from build123d import *

# Parameters (mm, degrees)
BOSS_EXTRUDE1_DEPTH = 46
CUT_EXTRUDE1_REACH  = 48
SKETCH2_R           = 1.65
SKETCH3_R           = 1.65
CUT_EXTRUDE2_DEPTH  = 5


with BuildPart() as part:
    # Sketch1 → Boss-Extrude1 (new body)
    with BuildSketch(Plane(origin=(-73, 0, 0), x_dir=(0, 0, 1), z_dir=(0, 1, 0))):
        Polygon((82, 10.55666667), (90, 8.18333333), (90, -9), (82, -9), align=None)
    extrude(amount=BOSS_EXTRUDE1_DEPTH)

    # Sketch2 → Cut-Extrude1 (cut, up to next)
    with BuildSketch(Plane.XZ, mode=Mode.PRIVATE) as cut_extrude1_sk1:
        with Locations((-73.41, 86)):
            Circle(SKETCH2_R)
    cut_extrude1_tool1 = extrude(cut_extrude1_sk1.sketch, amount=-CUT_EXTRUDE1_REACH, mode=Mode.PRIVATE) & part.part
    add(cut_extrude1_tool1.solids().sort_by_distance((-73.41, 0, 86))[0], mode=Mode.SUBTRACT)

    # Sketch3 → Cut-Extrude2 (cut)
    with BuildSketch(Plane.ZY.offset(82)):
        with Locations((86, 34.5)):
            Circle(SKETCH3_R)
        with Locations((86, 11.5)):
            Circle(SKETCH3_R)
    extrude(amount=-CUT_EXTRUDE2_DEPTH, mode=Mode.SUBTRACT)


solid = part.part
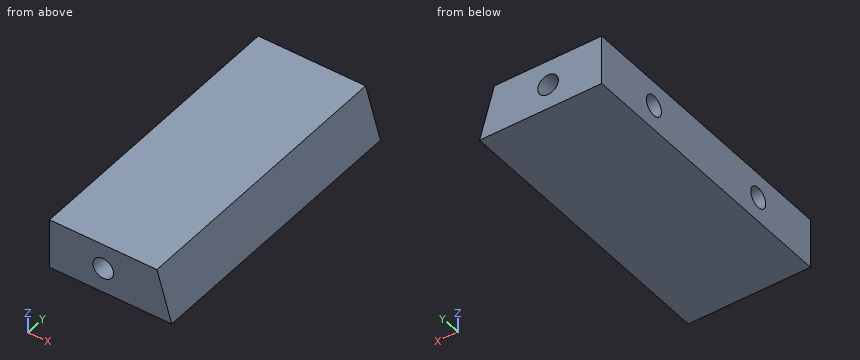
Part model, mm, in its own coordinate system. Coordinates: 2 decimals unless noted, no trailing zeros. Loops run counter-clockwise (first coordinate to the right, second up) from the corner with the lowest first, then second, coordinate; pieces in that order, holes last. Notation, with made-up numbers: (9, 37) -> (24, 37) arc R11 cw to (24, 43) -> close; hole circle Ø11 at (53, 55.25). An arc over 180 degrees is marked (long way). Use a Markdown table: item, result. Add a question column.
Item 1: Band-saw the part on C-C on x = -73.41. Write the cut outline in (y, z), plus the area to 3 significant figures.
Item 2: Band-saw the part on A-A on y = 11.5. Write the cut outline in (x, z).
Item 3: Probe probe 1 along Y at (x, z) = (-78.75, 86); probe 2 along Z at (x, y) = (-73.41, 22); probe 3 along Y at (x, z) = (-80.5, 87.25). List the from-to ranges inside material, lowest first.
Item 4: Band-saw the part on B-B on z = 86. Write the cut outline in (x, y).
Item 5: Band-saw the part on D-D on x = -79. Write the cut outline in (y, z), plus the area to 3 significant figures.
Item 6: Flat gauge pins, fed straight in: P1, Ø3, axis at y = 34.5, z = 86, coming from the +X side (3 decimals); P2, Ø4, axis at y = 37, z = 87, coming from the +X side; P3, Ø1.6, axis at y = 34, z = 85.5, coming from the -X side; P4, Ø2.5, axis at x = -73.41, z = 86, coming from the +Y side. Where does each tip first touch, or does it go through?
Geometry says:
| question | item | result |
|---|---|---|
| 1 | outline | (0, 82) -> (46, 82) -> (46, 84.35) -> (0, 84.35) -> close; (0, 87.65) -> (46, 87.65) -> (46, 90) -> (0, 90) -> close |
| 1 | area | 216 mm² |
| 2 | outline | (-82, 82) -> (-62.44, 82) -> (-64.82, 90) -> (-82, 90) -> (-82, 87.65) -> (-77, 87.65) -> (-77, 84.35) -> (-82, 84.35) -> close; hole circle Ø3.3 at (-73.41, 86) |
| 3 | probe 1 | 0 to 9.85, 13.15 to 32.85, 36.15 to 46 |
| 3 | probe 2 | 82 to 84.35, 87.65 to 90 |
| 3 | probe 3 | 0 to 10.42, 12.58 to 33.42, 35.58 to 46 |
| 4 | outline | (-82, 0) -> (-75.06, 0) -> (-75.06, 46) -> (-82, 46) -> (-82, 36.15) -> (-77, 36.15) -> (-77, 32.85) -> (-82, 32.85) -> (-82, 13.15) -> (-77, 13.15) -> (-77, 9.85) -> (-82, 9.85) -> close; (-71.76, 0) -> (-63.63, 0) -> (-63.63, 46) -> (-71.76, 46) -> close |
| 5 | outline | (0, 82) -> (46, 82) -> (46, 90) -> (0, 90) -> close; hole circle Ø3.3 at (11.5, 86); hole circle Ø3.3 at (34.5, 86) |
| 5 | area | 351 mm² |
| 6 | P1 | x = -63.185 |
| 6 | P2 | x = -63.33 |
| 6 | P3 | x = -77 |
| 6 | P4 | through |
